from build123d import *

# Parameters (mm, degrees)
F0_R     = 38.1
F1_DEPTH = 101.6
F2_DEPTH = 101.601
F3_DEPTH = 25.4
F5_DEPTH = 25.4
F6_R     = 25.4
F7_DEPTH = 38.1


with BuildPart() as f1:
    # F0 (on Front) → F1 (new body)
    with BuildSketch(Plane.XZ):
        Circle(F0_R)
        Polygon((3.91e-08, -19.2176233977), (-19.2176233977, -19.2176233977), (-19.2176233977, 0), (-19.2176233977, 19.2176233977), (2.72e-08, 19.2176233977), (19.2176233977, 19.2176233977), (19.2176233977, 0), (19.2176233977, -19.2176233977), align=None, mode=Mode.SUBTRACT)
        with BuildLine():
            ThreePointArc((2.72e-08, 19.2176233977), (13.5889118324, 13.5889118132), (19.2176233977, 0))
            Line((19.2176233977, 0), (19.2176233977, 19.2176233977))
            Line((19.2176233977, 19.2176233977), (2.72e-08, 19.2176233977))
        make_face()
        with BuildLine():
            ThreePointArc((-19.2176233977, 0), (-13.588911809, -13.5889118366), (3.91e-08, -19.2176233977))
            ThreePointArc((3.91e-08, -19.2176233977), (13.5889118366, -13.588911809), (19.2176233977, 0))
            ThreePointArc((19.2176233977, 0), (13.5889118324, 13.5889118132), (2.72e-08, 19.2176233977))
            ThreePointArc((2.72e-08, 19.2176233977), (-13.5889118132, 13.5889118324), (-19.2176233977, 0))
        make_face()
        with BuildLine():
            Line((-19.2176233977, 19.2176233977), (-19.2176233977, 0))
            ThreePointArc((-19.2176233977, 0), (-13.5889118132, 13.5889118324), (2.72e-08, 19.2176233977))
            Line((2.72e-08, 19.2176233977), (-19.2176233977, 19.2176233977))
        make_face()
        with BuildLine():
            Line((-19.2176233977, 0), (-19.2176233977, -19.2176233977))
            Line((-19.2176233977, -19.2176233977), (3.91e-08, -19.2176233977))
            ThreePointArc((3.91e-08, -19.2176233977), (-13.588911809, -13.5889118366), (-19.2176233977, 0))
        make_face()
        with BuildLine():
            ThreePointArc((19.2176233977, 0), (13.5889118366, -13.588911809), (3.91e-08, -19.2176233977))
            Line((3.91e-08, -19.2176233977), (19.2176233977, -19.2176233977))
            Line((19.2176233977, -19.2176233977), (19.2176233977, 0))
        make_face()
    extrude(amount=-F1_DEPTH)

    # F0 (on Front) → F2 (cut, through all)
    with BuildSketch(Plane.XZ):
        with BuildLine():
            ThreePointArc((-19.2176233977, 0), (-13.588911809, -13.5889118366), (3.91e-08, -19.2176233977))
            ThreePointArc((3.91e-08, -19.2176233977), (13.5889118366, -13.588911809), (19.2176233977, 0))
            ThreePointArc((19.2176233977, 0), (13.5889118324, 13.5889118132), (2.72e-08, 19.2176233977))
            ThreePointArc((2.72e-08, 19.2176233977), (-13.5889118132, 13.5889118324), (-19.2176233977, 0))
        make_face()
    extrude(amount=-F2_DEPTH, mode=Mode.SUBTRACT)

    # F0 (on Front) → F3 (cut)
    with BuildSketch(Plane.XZ):
        with BuildLine():
            ThreePointArc((19.2176233977, 0), (13.5889118366, -13.588911809), (3.91e-08, -19.2176233977))
            Line((3.91e-08, -19.2176233977), (19.2176233977, -19.2176233977))
            Line((19.2176233977, -19.2176233977), (19.2176233977, 0))
        make_face()
        with BuildLine():
            Line((-19.2176233977, 0), (-19.2176233977, -19.2176233977))
            Line((-19.2176233977, -19.2176233977), (3.91e-08, -19.2176233977))
            ThreePointArc((3.91e-08, -19.2176233977), (-13.588911809, -13.5889118366), (-19.2176233977, 0))
        make_face()
        with BuildLine():
            Line((-19.2176233977, 19.2176233977), (-19.2176233977, 0))
            ThreePointArc((-19.2176233977, 0), (-13.5889118132, 13.5889118324), (2.72e-08, 19.2176233977))
            Line((2.72e-08, 19.2176233977), (-19.2176233977, 19.2176233977))
        make_face()
        with BuildLine():
            ThreePointArc((2.72e-08, 19.2176233977), (13.5889118324, 13.5889118132), (19.2176233977, 0))
            Line((19.2176233977, 0), (19.2176233977, 19.2176233977))
            Line((19.2176233977, 19.2176233977), (2.72e-08, 19.2176233977))
        make_face()
    extrude(amount=-F3_DEPTH, mode=Mode.SUBTRACT)

    # F4 (on face) → F5 (cut)
    with BuildSketch(Plane(origin=(0, 101.6, 0), x_dir=(-1, 0, 0), z_dir=(0, 1, 0))):
        Polygon((-19.2176233977, 11.0953000419), (-19.2176233977, -11.0953000419), (0, -22.1906000837), (19.2176233977, -11.0953000419), (19.2176233977, 11.0953000419), (0, 22.1906000837), align=None)
    extrude(amount=-F5_DEPTH, mode=Mode.SUBTRACT)

    # F6 (on Right) → F7 (cut, symmetric)
    with BuildSketch(Plane.YZ):
        with Locations((53.5429239203, 0)):
            Circle(F6_R)
    extrude(amount=F7_DEPTH, both=True, mode=Mode.SUBTRACT)


solid = f1.part
Could you check a few things on this model? Use its own coordinates, in mm. A direction names the side the tool comes from. Coordinates: 2 decimals unless noted, no trailing zeros. Order: outer loops, then holes, each group sorted by start corner. A loop starts at its lowest first (then second) coordinate and runs counter-clockwise, first axis right, second up. Notation, with made-up numbers: (71.25, -31) - (99.25, -31) arc R18 cw to (99.25, -15) - close; hole circle Ø2 at (34, 89.25). An arc over 180 degrees is marked (long way). Answer in a Markdown table with one row per item. Add a question column.
(1) If we section it at C-C, the plane y = 19: Please give me the cut outline in (x, z), then the cut area to 3 significant figures.
(2) On a 3-axis mill with a long thin cutter (end or side, diameter ignored), from which of +Z, -Z, +X, -X, +Y, -Y can I reach the whole of each face in a straight line? I mean faces 1 (the face through (0, 13, 19.218)), 2 (the face through (0.532, 50.236, 25.184)), 3 (the face through (9.743, 89.078, -16.565)). Say none if no direction works.
(3) If we section it at A-A, the plane x = -32: Please give me the cut outline in (y, z).
(4) Will these pins go through, and if not, where does the flat tip stop? pin 1 (10 mm diameter, centred on x = 7, y = 51.5, fed in from -Z); pin 2 (6 mm diameter, centred on x = 7.5, z = -11, fed in from -Y); pin 3 (8 mm diameter, centred on y = 27, z = 7.5, fed in from -X); pin 4 (6.5 mm diameter, centred on y = 88.5, z = 4, fed in from +X).
(5) If we mould it in two halves opening along X, with no side actions, what happens to faces 4 (the face through (-28.08, 50.09, 25.75)), 5 (the face through (-1, 0, -25)), 6 (the face through (15, 25.4, 15))? For each: released by +X, released by -X, zero draft, split by the parting line, or undercut.
(6) I need wall thicknesses on L1, parallel to X at y = 13, z = 1; L2, parallel to Y at x = -34, z = 16; L3, parallel to Z at x = -14, y = 45. Which ranges of each line are inside material? Lowest first, please.
(7) If we section it at D-D, the plane x = 30: Please give me the cut outline in (y, z), then the cut area to 3 significant figures.
(8) If we section it at B-B, the plane z = -2.5: Please give me the cut outline in (x, y).
Results are:
| question | item | result |
|---|---|---|
| 1 | outline | circle Ø76.2 at (0, 0); hole (-19.22, -19.22) - (19.22, -19.22) - (19.22, 19.22) - (-19.22, 19.22) - close |
| 1 | area | 3,080 mm2 |
| 2 | face 1 | -Y |
| 2 | face 2 | +X, -X |
| 2 | face 3 | +Y |
| 3 | outline | (0, -20.68) - (38.79, -20.68) arc R25.4 cw to (38.79, 20.68) - (0, 20.68) - close; (68.29, -20.68) - (101.6, -20.68) - (101.6, 20.68) - (68.29, 20.68) arc R25.4 cw to start |
| 4 | pin 1 | stops at z = -38.05 |
| 4 | pin 2 | passes through |
| 4 | pin 3 | stops at x = -37.94 |
| 4 | pin 4 | stops at x = 38.09 |
| 5 | face 4 | split by the parting line |
| 5 | face 5 | zero draft |
| 5 | face 6 | undercut |
| 6 | L1 | x = -38.09 to -19.22, 19.22 to 38.09 |
| 6 | L2 | y = 0 to 33.82, 73.27 to 101.6 |
| 6 | L3 | z = -35.43 to -23.92, 23.92 to 35.43 |
| 7 | outline | (0, -23.49) - (43.87, -23.49) arc R25.4 cw to (43.87, 23.49) - (0, 23.49) - close; (63.22, -23.49) - (101.6, -23.49) - (101.6, 23.49) - (63.22, 23.49) arc R25.4 cw to start |
| 7 | area | 2,800 mm2 |
| 8 | outline | (-38.02, 0) - (-19.22, 0) - (-19.22, 25.4) - (-19.05, 25.4) - (-19.05, 28.27) - (-38.02, 28.27) - close; (-38.02, 78.82) - (-19.22, 78.82) - (-19.22, 101.6) - (-38.02, 101.6) - close; (19.05, 25.4) - (19.22, 25.4) - (19.22, 0) - (38.02, 0) - (38.02, 28.27) - (19.05, 28.27) - close; (19.22, 78.82) - (38.02, 78.82) - (38.02, 101.6) - (19.22, 101.6) - close |
